Autodesk Inventor part; units mm, degrees
ref_plane "Work Plane1" through (29, 0, 0) normal (0, -1, 0) x (1, 0, 0)
ref_plane "YZ Plane" through (0, 0, 0) normal (1, 0, 0) x (0, 1, 0)
ref_plane "XZ Plane" through (0, 0, 0) normal (0, 1, 0) x (-1, 0, 0)
sketch "Sketch1" plane through (0, 0, 0) normal (0, 0, 1) x (1, 0, 0)
  line L0 (-0.8667, 0) -> (14, 0)
  line L1 (14, 0) -> (14, 1.5)
  line L2 (14, 1.5) -> (0.5, 1.5)
  line L3 (0.5, 1.5) -> (0.1932, 1.5)
  line L4 (0.1932, 1.5) -> (0, 1.5)
  line L5 (0, 1.5) -> (0, 2.75)
  line L6 (0, 2.75) -> (-3, 2.75)
  line L7 (-3, 2.75) -> (-3, 1.4434)
  line L8 (-3, 1.4434) -> (-1.7, 1.4434)
  line L9 (-1.7, 1.4434) -> (-0.8667, 0)
  line L10 (-6.4, 0) -> (17.4, 0)
  line L11 (0, -0.55) -> (0, 3.3)
  line L12 (0.5, 1.5) -> (0, 1.5) construction
  dimension "d1" = 13.5
  dimension "d2" = 0.3068
  dimension "d3" = 3
  dimension "d4" = 1.3
  dimension "d5" = 60
  dimension "d6" = 3
  dimension "d7" = 3
  dimension "d8" = 2.8868
  dimension "d9" = 5.5
  dimension "d26" = 14
revolve "Body" add sketch "Sketch1" angle 360 about axis through (-0.8667, 0, 0) along (1, 0, 0)
sketch "Sketch2" plane through (-3, 0, 0) normal (-1, 0, 0) x (0, 0, 1)
  circle A0 centre (0, 0) radius 1.4434
  line L0 (0, -3.85) -> (0, 3.85)
  line L1 (-3.85, 0) -> (3.85, 0)
  line L2 (1.4434, 0) -> (0.7217, -1.25)
  line L3 (0.7217, -1.25) -> (-0.7217, -1.25)
  line L4 (-0.7217, -1.25) -> (-1.4434, 0)
  line L5 (-1.4434, 0) -> (-0.7217, 1.25)
  line L6 (-0.7217, 1.25) -> (0.7217, 1.25)
  line L7 (0.7217, 1.25) -> (1.4434, 0)
extrude "Slot" add sketch "Sketch2" against normal up to next contours L7 A0 | A0 L2 | L6 L0 A0 | A0 L0 L3 | L0 L6 A0 | A0 L3 L0 | L4 A0 | A0 L5
fillet "Fillet1" radius 0.3 1 edges at (-3, -2.75, 0)
thread "Thread"
chamfer "Chamfer1" distance 0.3067 distance2 0.3067 1 edges at (14, -1.5, 0) measured on face at (14, -0.6587, -0.1791)
ref_plane "Work Plane1" through (29, 0, 0) normal (0, -1, 0) x (1, 0, 0)
fillet "Fillet2" radius 0.1 1 edges at (0, -1.5, 0)
equation "\"d1\" = GEL"
equation "\"d3\" = KOH"
equation "\"d4\" = INTI"
equation "\"d6\" = GD"
equation "\"d7\" = BDM"
equation "\"d8\" = 1.1547 * SW"
equation "\"d9\" = KOD"
equation "\"d26\" = NLG"
equation "\"d30\" = R"
equation "\"d17\" = RR"
equation "\"d13\" = GEL"
equation "\"d15\" = -0.5 * SPD + 0.5 * GD"
equation "\"d16\" = GUL"
equation "\"GD\" = NND"
equation "\"NLG\" = 14"
equation "\"GEL\" = 13.5"
equation "\"KOD\" = 5.5"
equation "\"KOH\" = NND"
equation "\"INTI\" = 1.3"
equation "\"GAL\" = 0.61345 * PTC"
equation "\"GUL\" = 0.61345 * PTC"
equation "\"BDM\" = NND"
equation "\"SW\" = 2.5"
equation "\"RR\" = 0.3"
equation "\"SPD\" = NND - 1.2269 * PTC"
equation "\"R\" = 0.1"
equation "\"TOA\" = 30deg"
equation "\"GD1\" = THREADDIA - 1.2269 * PTC"
equation "\"THREADDIA\" = 3"
equation "\"FAWI\" = 45deg"
equation "\"PTC\" = 0.5"
equation "\"NND\" = 3"
equation "\"E0\" = 1.155 * SW"
properties part number "Screw GB/T 70.1 M3 x 14" material "Steel, Mild"
Geometry check sheet. Reference: the model listing, model coordinates, mm. A direction names the side the tool comes from. Give positions to 0.01 mm unless a question says otherwise; leave off trailing zeros. Loops run counter-clockwise (first coordinate to the right, second up) from the corner with the lowest first, then second, coordinate; pieces in that order, holes last. Notation, with made-up numbers: (-27.75, -38.5) -> (26.25, -38.5) arc R13 cw to (26.25, -16.5) -> close; hole circle Ø4 at (20, -1.5). An arc over 180 degrees is marked (long way). Answer in a Markdown table with one row per item. Add a question column.
1) Gauge pin test, flat ends, axial feed: P1, Ø1, axis at x = 10.5, z = -1.5, coming from the +Y side; P2, Ø2, axis at x = 4.5, z = -1.5, coming from the +Y side. Record the tip position at first contact, or that the pin passes through.
2) Draft check along Y on faces 3 (the face through (-2.304, -0.616, 1.088)), 4 (the face through (0, 2, 0)), 5 (the face through (6.8, -1.5, -0.07)). Enter one of: pulls with the +Y half, pulls with the -Y half, needs draft (parallel to the pull), parting line crosses it, or undercut.
3) Material ranges on probe 1 along X at (y, z) = (-1, 2.25); probe 2 along Z at (x, y) = (3.5, -0.1); probe 3 along X at (y, z) = (-0.6, -0.7), recorded low to high. Write a range as from..to.
4) Cross-section at A-A on x = 2. Record the boundary of the cut face in (y, z), and give its area (3 significant figures).
5) Set-up check for faces 1 (the face through (-3, -1.1, 1.1)), 2 (the face through (-2.3, 0.63, 1.08)): record each of +Z, -Z, +X, -X, +Y, -Y from which the full face is reachable in a straight line by a thin tool's end or side.
Outcome:
| question | item | result |
|---|---|---|
| 1 | P1 | stops at y = 1.12 |
| 1 | P2 | stops at y = 1.41 |
| 2 | face 3 | undercut |
| 2 | face 4 | needs draft |
| 2 | face 5 | parting line crosses it |
| 3 | probe 1 | x = -3..0 |
| 3 | probe 2 | z = -1.5..1.5 |
| 3 | probe 3 | x = -1.4..14 |
| 4 | outline | circle Ø3 at (0, 0) |
| 4 | area | 7.07 mm^2 |
| 5 | face 1 | +Z, -Z, -X, +Y, -Y |
| 5 | face 2 | -X |
